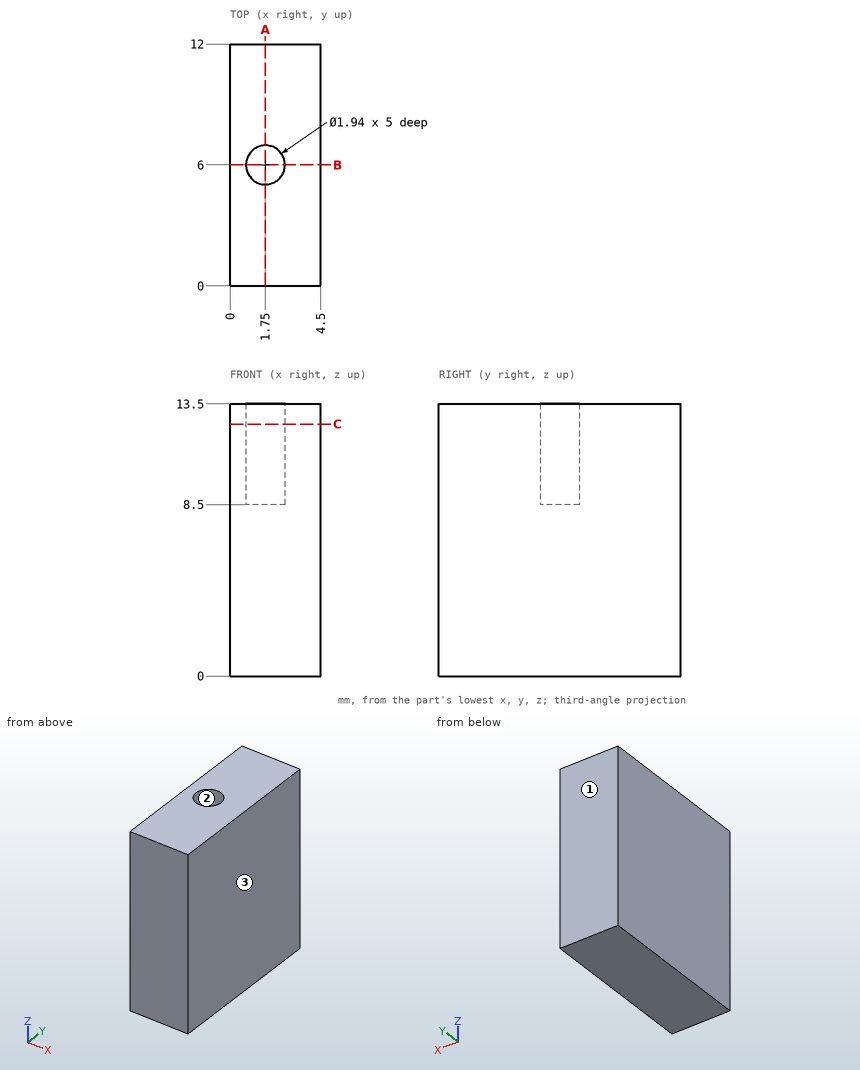
Source: three-view drawing plus pictorial views. Frame: mm from the lowest corner of the part. Give positions to 0.01 mm unless a question says otherwise; leave off trailing zeros. Loops run counter-clockwise (first coordinate to the right, second up) from the corner with the lowest first, then second, coordinate; pieces in that order, holes last.
1) Section query A-A on x = 1.75. Return the cut outline in (y, z).
A:
outline: (0, 0) - (12, 0) - (12, 13.5) - (6.97, 13.5) - (6.97, 8.5) - (5.03, 8.5) - (5.03, 13.5) - (0, 13.5) - close
2) Section query B-B on y = 6. Return the cut outline in (x, z).
A:
outline: (0, 0) - (4.5, 0) - (4.5, 13.5) - (2.72, 13.5) - (2.72, 8.5) - (0.78, 8.5) - (0.78, 13.5) - (0, 13.5) - close
3) Line query: L1, parallel to Y at x = 1.75, z = 10.2; L2, parallel to Z at x = 1.6, y = 5.5. Output: solid intervals per line, ascending.
A:
L1: y = 0 to 5.03, 6.97 to 12
L2: z = 0 to 8.5
4) Mould query, pull axis Y, two halves, no side actions, for the marked faces 1, 2 and 3. Classes: released by +Y, released by -Y, zero draft, split by the parting line, or undercut.
A:
face 1: released by +Y
face 2: undercut
face 3: zero draft
5) Section query C-C on z = 12.5. Return the cut outline in (x, y).
A:
outline: (0, 0) - (4.5, 0) - (4.5, 12) - (0, 12) - close; hole circle Ø1.94 at (1.75, 6)
